from build123d import *

# Parameters (mm, degrees)
F1_W     = 51.75
F1_H     = 20
F2_DEPTH = 7.5
F3_W     = 5
F3_H     = 71.75
F4_DEPTH = 7.5
F0_R     = 6.75
F5_DEPTH = 3.4
F6_DEPTH = 20
F7_R     = 3.2
F8_DEPTH = 25


with BuildPart() as f2:
    # F1 (on Top) → F2 (new body)
    with BuildSketch(Plane.XY):
        Polygon((13.25, 65), (-6.75, 65), (-6.75, -6.75), (13.25, -6.75), (13.25, 13.25), align=None)
        Polygon((65, 13.25), (13.25, 65), (13.25, 13.25), align=None)
        with Locations((39.125, 3.25)):
            Rectangle(F1_W, F1_H)
    extrude(amount=-F2_DEPTH)

    # F3 (on face) → F4 (join)
    with BuildSketch(Plane.XY):
        with Locations((-9.25, 29.125)):
            Rectangle(F3_W, F3_H)
        Polygon((65, -6.75), (-6.75, -6.75), (-11.75, -6.75), (-11.75, -11.75), (65, -11.75), align=None)
    extrude(amount=-F4_DEPTH)

    # F0 (on Top) → F5 (cut)
    with BuildSketch(Plane.XY):
        with Locations((55, 0)):
            Circle(F0_R)
        with Locations((25, 0)):
            Circle(F0_R)
        with Locations((0, 25)):
            Circle(F0_R)
        with Locations((0, 55)):
            Circle(F0_R)
    extrude(amount=-F5_DEPTH, mode=Mode.SUBTRACT)

    # F3 (on face) → F6 (join)
    with BuildSketch(Plane.XY):
        with Locations((-9.25, 29.125)):
            Rectangle(F3_W, F3_H)
        Polygon((65, -6.75), (-6.75, -6.75), (-11.75, -6.75), (-11.75, -11.75), (65, -11.75), align=None)
    extrude(amount=F6_DEPTH)

    # F7 (on face) → F8 (cut)
    with BuildSketch(Plane.XY):
        with Locations((0, 25)):
            Circle(F7_R)
        with Locations((0, 55)):
            Circle(F7_R)
        with Locations((25, 0)):
            Circle(F7_R)
        with Locations((55, 0)):
            Circle(F7_R)
    extrude(amount=-F8_DEPTH, mode=Mode.SUBTRACT)


solid = f2.part
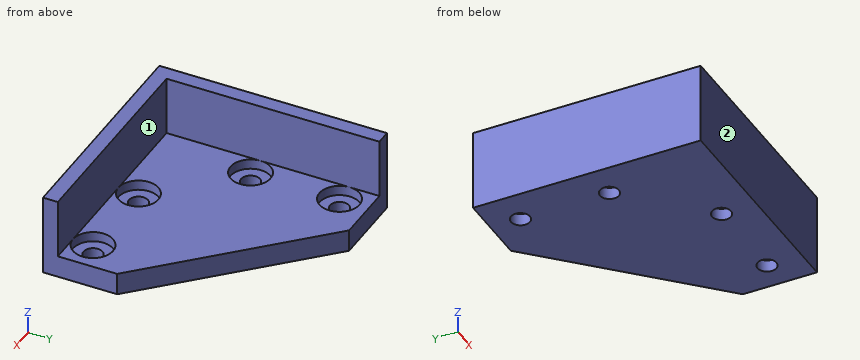
Build history of the part. All positions in model axes, mm. Face numbers are marked on the shaded views. A direction names the side the tool comes from. Round coordinates to 2 decimals unless told otherwise and drop trailing zeros. Write each loop counter-clockwise with the first axis right and the second up, starting at its lowest first coordinate (ties: lowest second). Pieces come first, ordered by that corner, then holes. Notation, with made-up numbers: (-35.75, 76.25) -> (6.25, 76.25) arc R32 ccw to (6.25, 110.25) -> close; hole circle Ø11 at (26.25, 84). An arc over 180 degrees is marked (long way). Use one line per item in the form item = value.
Q1. Band-saw the part on B-B, the plane z = -1. Write the cut outline in (x, y).
Conclusion:
outline = (-11.75, -11.75) -> (65, -11.75) -> (65, 13.25) -> (13.25, 65) -> (-11.75, 65) -> close; hole circle Ø13.5 at (0, 25); hole circle Ø13.5 at (0, 55); hole circle Ø13.5 at (25, 0); hole circle Ø13.5 at (55, 0)
Q2. Band-saw the part on A-A, the plane x = 0. Write the cut outline in (y, z).
Conclusion:
outline = (-11.75, -7.5) -> (21.8, -7.5) -> (21.8, -3.4) -> (18.25, -3.4) -> (18.25, 0) -> (-6.75, 0) -> (-6.75, 20) -> (-11.75, 20) -> close; (28.2, -7.5) -> (51.8, -7.5) -> (51.8, -3.4) -> (48.25, -3.4) -> (48.25, 0) -> (31.75, 0) -> (31.75, -3.4) -> (28.2, -3.4) -> close; (58.2, -7.5) -> (65, -7.5) -> (65, 0) -> (61.75, 0) -> (61.75, -3.4) -> (58.2, -3.4) -> close
Q3. Band-saw the part on C-C, the plane y = 37.5. Write the cut outline in (x, z), then the cut area to 3 significant figures.
Conclusion:
outline = (-11.75, -7.5) -> (40.75, -7.5) -> (40.75, 0) -> (-6.75, 0) -> (-6.75, 20) -> (-11.75, 20) -> close
area = 494 mm²
Q4. Band-saw the part on D-D, the plane x = 53. Write the cut outline in (y, z).
Conclusion:
outline = (-11.75, -7.5) -> (-2.5, -7.5) -> (-2.5, -3.4) -> (-6.45, -3.4) -> (-6.45, 0) -> (-6.75, 0) -> (-6.75, 20) -> (-11.75, 20) -> close; (2.5, -7.5) -> (25.25, -7.5) -> (25.25, 0) -> (6.45, 0) -> (6.45, -3.4) -> (2.5, -3.4) -> close
Q5. Tool access for the marked faces 1 and 2: list every direction of +Z, -Z, +X, -X, +Y, -Y with a clear straight run to the whole face (end or side of a thin tool).
Conclusion:
face_1 = +Z, +X, +Y
face_2 = +Z, -Z, +X, -X, -Y
Q6. Drill centre lines: L1, parallel to X at y = 0, z = -1.4; L2, parallel to Y at x = 0, z = -5.6. Where is each one in solid material? Low to high.
Conclusion:
L1 = -11.75 to 18.25, 31.75 to 48.25, 61.75 to 65
L2 = -11.75 to 21.8, 28.2 to 51.8, 58.2 to 65
Q7. Drop flat-ended pins along their axis: P1, Ø10, axis at x = 0, y = 25, coming from the +Z side; P2, Ø7, axis at x = 22, y = 1.5, coming from the +Z side; P3, Ø5, axis at x = 0, y = 55, coming from the +Z side; P4, Ø10, axis at y = 38.5, z = 14.5, coming from the +X side. Give the stop position or say it passes through.
Conclusion:
P1 = -3.4
P2 = 0
P3 = through
P4 = -6.75
